Verification items for the finished model (mm, model axes). A direction names the side the tool comes from. Coordinates: 2 decimals unless noted, no trailing zeros. Order: outer loops, then holes, each group sorted by start corner. A loop starts at its lowest first (then second) coordinate and runs counter-clockwise, first axis right, second up. Notation, with made-up numbers: M 47.5,-31.5 L 78.5,-31.5 A19 ccw 78.5,-9.5 Z; hole C 32.25,-17.5 d5. An arc over 180 degrees is marked long. Return JSON: item names as keys, results as strings. Group by question number.
1. Section check A-A, the plane y = 10.5. Record the cut outline in (x, z).
2. Gauge pin test, flat end, axial feed: pin 1 (2.5 mm diameter, centred on x = -2, z = 1.5, fed in from +Y). Record the tip position at first contact, or that the pin passes through.
3. Mould release check, pull along Z, two halves, no side actions. Record for faces 3 (the flat face through (0, 12, 6)), 4 (the flat face through (0, 6, 6.5)), 5 (the flat face through (0, 6, -6.5)), 6 (the cylindrical face through (-3.756, 3.944, -3.293)): +Z half, -Z half, draft (parallel to the pull), parting line (faces both ways), or undercut.
4. Material ranges on line 1 along X through (y, z) = (5, 2.5) (3 decimals); line 2 along Z through (x, y) = (-2.75, 5.75); line 3 along Z through (x, y) = (4, 10.75), recorded low to high.
5. Section check C-C, the plane y = 7.25. Give the number of separate pieces and of enclosed holes in the cut face, plus the area to 3 significant figures.
6. Section check B-B, the plane x = -5. Record the cut outline in (y, z) (3 decimals), plus the area to 3 significant figures.
7. Set-up check for faces 1 (the flat face through (0, 6, -4.5)), 2 (the cylindrical face through (6.244, 3.944, 1.707)): record each of +Z, -Z, +X, -X, +Y, -Y from which the full face is reachable in a straight line by a thin tool's end or side.
8. Section check D-D, the plane z = 2.5. Record the cut outline in (x, y) (3 decimals), plus the area to 3 significant figures.
```python
from build123d import *

# Parameters (mm, degrees)
SKETCH1_W            = 15
SKETCH1_H            = 13
BOSS_EXTRUDE1_DEPTH  = 8
SKETCH8_W            = 15
SKETCH8_H            = 1.5
BOSS_EXTRUDE4_DEPTH  = 4
SKETCH9_W            = 15
SKETCH9_H            = 0.5
CUT_EXTRUDE3_DEPTH   = 4
CHAMFER1_SIZE        = 0.4
SKETCH4_R            = 1.475
CUT_EXTRUDE2_DEPTH   = 8
LPATTERN1_COUNT      = 3
LPATTERN1_PITCH      = 5
LPATTERN1_COUNT_DIR2 = 2
LPATTERN1_PITCH_DIR2 = 5


with BuildPart() as part:
    # Sketch1 → Boss-Extrude1 (new body)
    with BuildSketch(Plane(origin=(0, 0, 0), x_dir=(1, 0, 0), z_dir=(0, 1, 0))):
        Rectangle(SKETCH1_W, SKETCH1_H)
    extrude(amount=BOSS_EXTRUDE1_DEPTH)

    # Sketch8 → Boss-Extrude4 (add)
    with BuildSketch(Plane(origin=(0, 8, 0), x_dir=(1, 0, 0), z_dir=(0, 1, 0))):
        with Locations((0, 5.75)):
            Rectangle(SKETCH8_W, SKETCH8_H)
        with Locations((0, -5.75)):
            Rectangle(SKETCH8_W, SKETCH8_H)
    extrude(amount=BOSS_EXTRUDE4_DEPTH)

    # Sketch9 → Cut-Extrude3 (cut)
    with BuildSketch(Plane(origin=(0, 8, 0), x_dir=(1, 0, 0), z_dir=(0, 1, 0))):
        with Locations((0, 4.75)):
            Rectangle(SKETCH9_W, SKETCH9_H)
        with Locations((0, -4.75)):
            Rectangle(SKETCH9_W, SKETCH9_H)
    extrude(amount=-CUT_EXTRUDE3_DEPTH, mode=Mode.SUBTRACT)

    # Chamfer1
    chamfer1_edges = [part.edges().sort_by_distance(p)[0] for p in [
        (0, 4, -5),
        (0, 4, 5),
    ]]
    chamfer(chamfer1_edges, length=CHAMFER1_SIZE)

    # Sketch4 → Cut-Extrude2 (cut)
    with BuildSketch(Plane.XZ):
        with Locations(Location((-5, 2.5, 0), (0, 0, 270))):
            Circle(SKETCH4_R)
    cut_extrude2 = extrude(amount=-CUT_EXTRUDE2_DEPTH, mode=Mode.SUBTRACT)

    # LPattern1: Cut-Extrude2 3 × 2
    with Locations(*[(i * LPATTERN1_PITCH, 0, -j * LPATTERN1_PITCH_DIR2) for i in range(LPATTERN1_COUNT) for j in range(LPATTERN1_COUNT_DIR2) if (i, j) != (0, 0)]):
        add(cut_extrude2, mode=Mode.SUBTRACT)


solid = part.part
```
Answers follow:
{
 "1": {"outline": "M -7.5,-6.5 L 7.5,-6.5 L 7.5,-5 L -7.5,-5 Z; M -7.5,5 L 7.5,5 L 7.5,6.5 L -7.5,6.5 Z"},
 "2": {"pin 1": "y = 8"},
 "3": {"face 3": "draft", "face 4": "+Z half", "face 5": "-Z half", "face 6": "undercut"},
 "4": {"line 1": "-7.5 to -6.475, -3.525 to -1.475, 1.475 to 3.525, 6.475 to 7.5", "line 2": "-6.5 to -5, -4.5 to 4.5, 5 to 6.5", "line 3": "-6.5 to -5, 5 to 6.5"},
 "5": {"separate pieces": "3", "enclosed holes": "6", "area": "139 mm^2"},
 "6": {"outline": "M 0,-6.5 L 12,-6.5 L 12,-5 L 4.4,-5 L 4,-4.6 L 4,-4.5 L 8,-4.5 L 8,-3.975 L 0,-3.975 Z; M 0,-1.025 L 8,-1.025 L 8,1.025 L 0,1.025 Z; M 0,3.975 L 8,3.975 L 8,4.5 L 4,4.5 L 4,4.6 L 4.4,5 L 12,5 L 12,6.5 L 0,6.5 Z", "area": "65.0 mm^2"},
 "7": {"face 1": "+X, -X, +Y", "face 2": "+Y, -Y"},
 "8": {"outline": "M -7.5,0 L -6.475,0 L -6.475,8 L -7.5,8 Z; M -3.525,0 L -1.475,0 L -1.475,8 L -3.525,8 Z; M 1.475,0 L 3.525,0 L 3.525,8 L 1.475,8 Z; M 6.475,0 L 7.5,0 L 7.5,8 L 6.475,8 Z", "area": "49.2 mm^2"}
}
